Part print with two shaded views. Sizes in mm from the minimum x, y, z corner. Give positions to 0.01 mm unless a question says otherwise; leave off trailing zeros. Loops run counter-clockwise (first coordinate to the right, second up) from the corner with the lowest first, then second, coordinate; pieces in that order, holes last. Notation, with made-up numbers: M -4.75,-34 L 53.25,-34 A23 ccw 53.25,0 Z; hole C 86.5,-2.75 d11. An arc over 180 degrees is marked long. Answer in a Markdown table with one row per item.
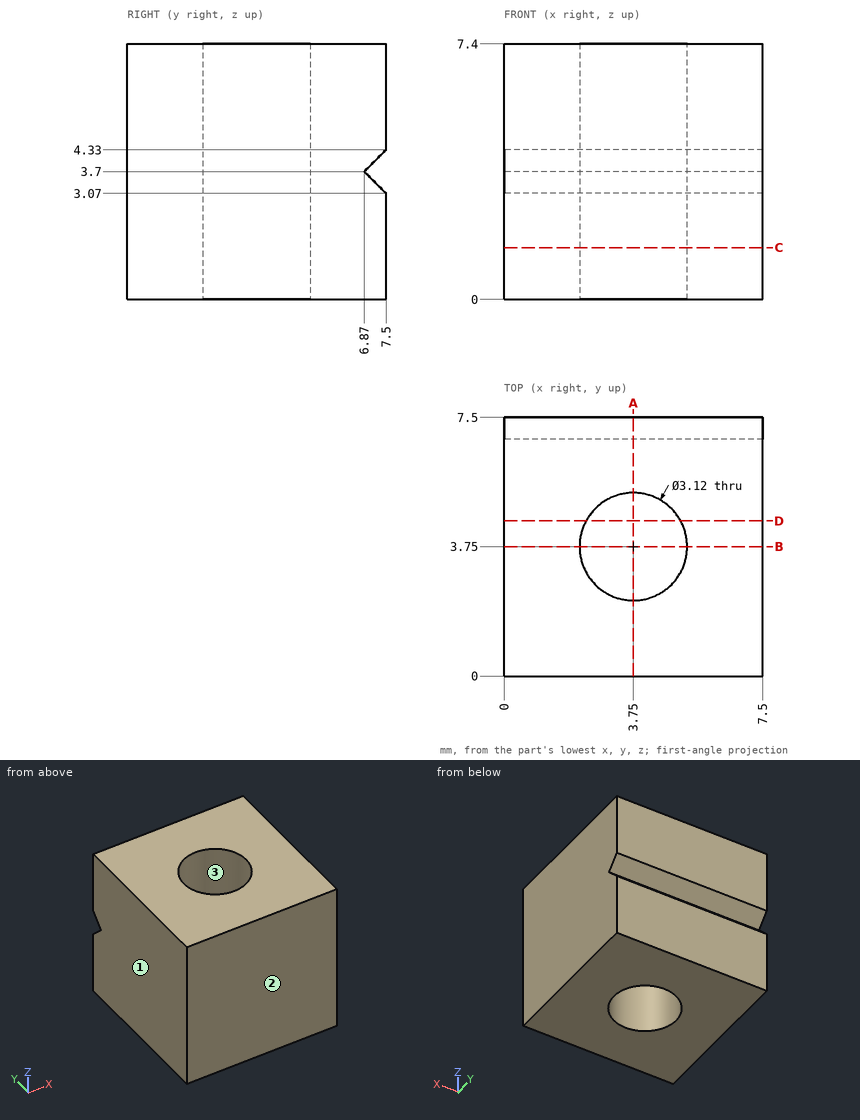
Q1. Saw through at A-A (x = 3.75). Give the cut face in (y, z).
Reported:
| item | result |
|---|---|
| outline | M 0,0 L 2.19,0 L 2.19,7.4 L 0,7.4 Z; M 5.31,0 L 7.5,0 L 7.5,3.07 L 6.87,3.7 L 7.5,4.33 L 7.5,7.4 L 5.31,7.4 Z |
Q2. Probe probe 1 along Y at (x, z) = (3.75, 2.5); probe 2 along X at (y, z) = (2.75, 5.75); probe 3 along X at (y, z) = (3.5, 1.75). List the from-to ranges inside material, lowest first.
Reported:
| item | result |
|---|---|
| probe 1 | 0 to 2.19, 5.31 to 7.5 |
| probe 2 | 0 to 2.55, 4.95 to 7.5 |
| probe 3 | 0 to 2.21, 5.29 to 7.5 |
Q3. Mould opens along Y. For the marked faces 1, 2 and 3 say: released by +Y, released by -Y, zero draft, split by the parting line, or undercut.
Reported:
| item | result |
|---|---|
| face 1 | zero draft |
| face 2 | released by -Y |
| face 3 | undercut |
Q4. Saw through at C-C (z = 1.5). Give the cut face in (x, y), and give its area (3 significant figures).
Reported:
| item | result |
|---|---|
| outline | M 0,0 L 7.5,0 L 7.5,7.5 L 0,7.5 Z; hole C 3.75,3.75 d3.12 |
| area | 48.6 mm² |
Q5. Saw through at B-B (y = 3.75). Give the cut face in (x, z), and give its area (3 significant figures).
Reported:
| item | result |
|---|---|
| outline | M 0,0 L 2.19,0 L 2.19,7.4 L 0,7.4 Z; M 5.31,0 L 7.5,0 L 7.5,7.4 L 5.31,7.4 Z |
| area | 32.4 mm² |
Q6. Saw through at D-D (y = 4.5). Give the cut face in (x, z).
Reported:
| item | result |
|---|---|
| outline | M 0,0 L 2.38,0 L 2.38,7.4 L 0,7.4 Z; M 5.12,0 L 7.5,0 L 7.5,7.4 L 5.12,7.4 Z |
Q7. Drop a flat-ended pin along its axis: pin 1 (4 mm diameter, centred on x = 6.5, z = 5.5, fed in from -Y). Give the stop position or say it passes through.
Reported:
| item | result |
|---|---|
| pin 1 | y = 0 |
